The drawing under review shows one solid part. Ordinate dimensions are in mm from its lowest x, y, z. A direction names the side the tool comes from. Round coordinates to 2 decimals unless told otherwise and drop trailing zeros. Order: outer loops, then holes, each group sorted by start corner. A loop starts at its lowest first (then second) coordinate and runs counter-clockwise, first axis right, second up. Notation, with made-up numbers: (85, 70.25) -> (107, 70.25) arc R7 cw to (107, 83.25) -> close; hole circle Ø4 at (32.5, 4). An arc over 180 degrees is marked (long way). Use a Markdown table: item, result. Add a question column.
1) Wall thickness on line 1 along Z through (x, y) = (43.5, 20); line 2 along Z through (x, y) = (44.45, 34.5) (3 decimals); line 3 along X through (y, z) = (8.5, 92): over which ranges is each line inside the solid? List them lowest first. Write a range as [from, to].
2) Consider section D-D (x = 61). State the section outline as (y, z) points.
3) Consider section C-C (z = 51). State the section outline as (x, y) points, plus the area to 3 significant figures.
4) Consider section A-A (y = 10). State the section outline as (x, z) points, plus the area to 3 significant figures.
5) Draft analysis for pull direction X (two halves, no side actions). For the marked faces 4, 5 and 6, state which applies: pulls with the +X half, pulls with the -X half, needs draft (parallel to the pull), parting line crosses it, or undercut.
6) Clearance check with flat-ended pins moving along their axes: P1, Ø14, axis at y = 52.5, z = 49, coming from the -X side; P2, Ø9.5, axis at x = 80.5, z = 109.5, coming from the +Y side; P3, Ø4, axis at y = 50.5, z = 75, coming from the +X side. State where each tip first meets the part, or that it passes through.
7) Machinability: for the marked faces 1, 2 and 3, which of the approach directions +Z, -Z, +X, -X, +Y, -Y give a long, thin tool a straight path to every point of the face, cutting with its end or side? Answer none if there is none.
8) Consider section B-B (x = 44.45). State the section outline as (y, z) points (3 decimals).
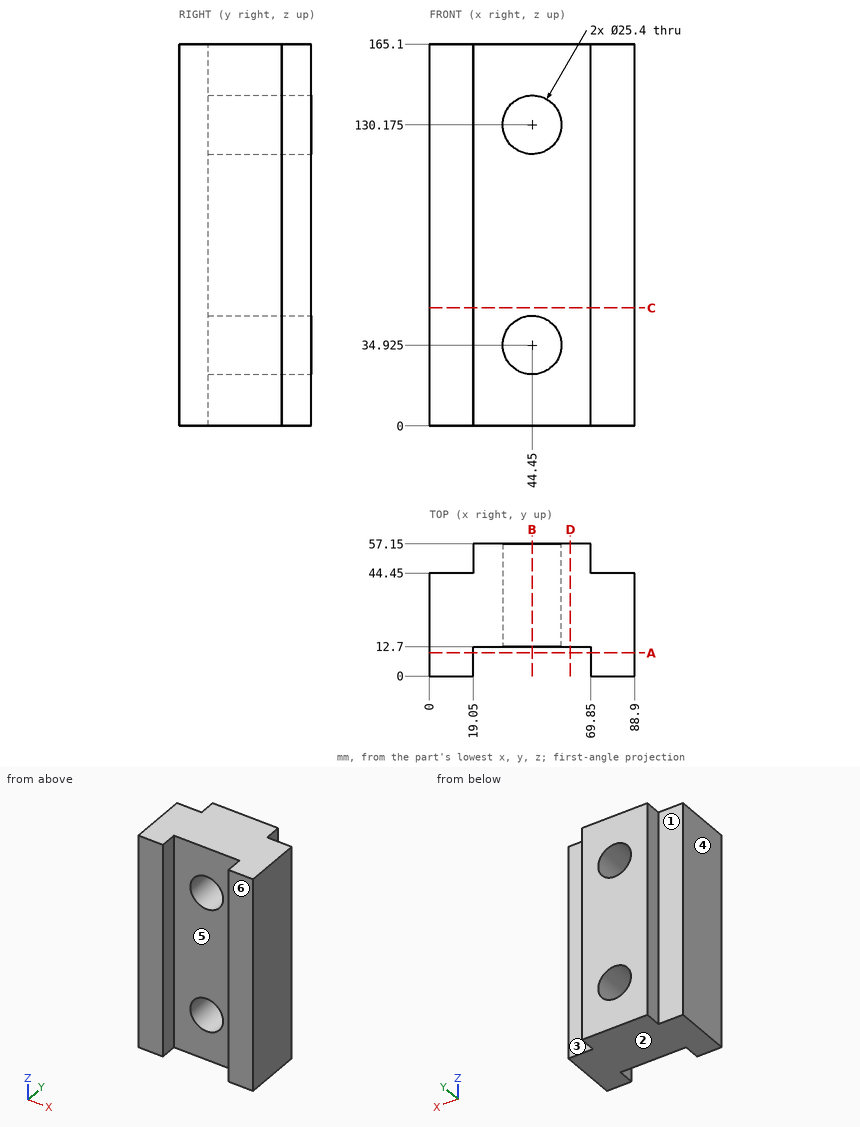
Results list:
| question | item | result |
|---|---|---|
| 1 | line 1 | [0, 22.26], [47.59, 117.51], [142.84, 165.1] |
| 1 | line 2 | [0, 22.225], [47.625, 117.475], [142.875, 165.1] |
| 1 | line 3 | [0, 19.05], [69.85, 88.9] |
| 2 | outline | (12.7, 0) -> (57.15, 0) -> (57.15, 165.1) -> (12.7, 165.1) -> close |
| 3 | outline | (0, 0) -> (19.05, 0) -> (19.05, 12.7) -> (69.85, 12.7) -> (69.85, 0) -> (88.9, 0) -> (88.9, 44.45) -> (69.85, 44.45) -> (69.85, 57.15) -> (19.05, 57.15) -> (19.05, 44.45) -> (0, 44.45) -> close |
| 3 | area | 3,950 mm2 |
| 4 | outline | (0, 0) -> (19.05, 0) -> (19.05, 165.1) -> (0, 165.1) -> close; (69.85, 0) -> (88.9, 0) -> (88.9, 165.1) -> (69.85, 165.1) -> close |
| 4 | area | 6,290 mm2 |
| 5 | face 4 | pulls with the -X half |
| 5 | face 5 | undercut |
| 5 | face 6 | needs draft |
| 6 | P1 | x = 19.05 |
| 6 | P2 | y = 44.45 |
| 6 | P3 | x = 69.85 |
| 7 | face 1 | +Z, -Z, -X, +Y |
| 7 | face 2 | -Z, +X, -X, +Y, -Y |
| 7 | face 3 | +Z, -Z, +X, +Y |
| 8 | outline | (12.7, 0) -> (57.15, 0) -> (57.15, 22.225) -> (12.7, 22.225) -> close; (12.7, 47.625) -> (57.15, 47.625) -> (57.15, 117.475) -> (12.7, 117.475) -> close; (12.7, 142.875) -> (57.15, 142.875) -> (57.15, 165.1) -> (12.7, 165.1) -> close |
